Autodesk Inventor part; units mm, degrees
ref_plane "YZ Plane" through (0, 0, 0) normal (1, 0, 0) x (0, 1, 0)
ref_plane "XZ Plane" through (0, 0, 0) normal (0, 1, 0) x (-1, 0, 0)
ref_plane "XY Plane" through (0, 0, 0) normal (0, 0, 1) x (1, 0, 0)
sketch "Sketch1" plane through (0, 0, 0) normal (0, 1, 0) x (-1, 0, 0)
  circle A0 centre (0, 0) radius 3.1369
  dimension "d0" = 6.2738
extrude "Extrusion1" add sketch "Sketch1" along normal mid plane 6.35
sketch "Sketch2" plane through (0, 3.175, 0) normal (0, 1, 0) x (1, 0, 0)
  circle A0 centre (0, 0) radius 4.699
  dimension "d3" = 9.398
extrude "Extrusion2" add sketch "Sketch2" along normal blind 6.35
sketch "Sketch3" plane through (0, -3.175, 0) normal (0, -1, 0) x (1, 0, 0)
  circle A0 centre (0, 0) radius 3.1369
extrude "Extrusion3" add sketch "Sketch3" along normal blind 12.7
thread "Thread1"
sketch "Sketch4" plane through (0, 9.525, 0) normal (0, 1, 0) x (1, 0, 0)
  line L0 (0, -3.6955) -> (-3.2004, -1.8478)
  line L1 (-3.2004, -1.8478) -> (-3.2004, 1.8478)
  line L2 (-3.2004, 1.8478) -> (0, 3.6955)
  line L3 (0, 3.6955) -> (3.2004, 1.8478)
  line L4 (3.2004, 1.8478) -> (3.2004, -1.8478)
  line L5 (3.2004, -1.8478) -> (0, -3.6955)
  point P0 (0, 0)
  point P1 (0, 0)
  dimension "d10" = 6.4008
extrude "Extrusion4" cut sketch "Sketch4" against normal blind 3.81
properties part number "Bolt 2.0" material "Steel, Galvanized"
The listing builds one solid part. Answer for the finished solid, in the listing's coordinates (mm). A direction names the side the tool comes from. Give positions to 0.01 mm unless a question says otherwise; leave off trailing zeros. Write each loop counter-clockwise with the first axis right and the second up, starting at its lowest first coordinate (ties: lowest second). Pieces come first, ordered by that corner, then holes.
Item 1: Section A-A, the plane x = 2.25 is taken. Write down the section's boundary in (y, z) (1 decimal), plus the area to 3 significant figures.
Item 2: Section C-C, the plane y = 5 is taken. Write down the section's boundary in (x, z), plus the area to 3 significant figures.
Item 3: Determine the mould class of faces 4 (the flat face through (0, -15.875, 0)), 5 (the cylindrical face through (-0.61, 6.31, 4.66)), 6 (the flat face through (-1.578, 7.647, 2.785)) for opening direction Z: released by +Z, released by -Z, zero draft, split by the parting line, or undercut.
Item 4: Section B-B, the plane z = 0.75 is taken. Write down the section's boundary in (x, y) (3 decimals).
Item 5: Which of the six approach directions +Z, -Z, +X, -X, +Y, -Y give full straight-line access (tool end or side, diameter ignored) to faces 1 (the flat face through (1.578, 7.647, -2.785)), 2 (the flat face through (2, 9.525, 3)), 3 (the flat face through (-1.1, 3.175, 3.1))?
Item 6: Section D-D, the plane y = -12.75 is taken. Write down the section's boundary in (x, z), plus the area to 3 significant figures.
Item 7: Flat-ended cylindrical pins translate along their axes: P1, Ø1.9, axis at x = -1.5, z = 1.5, coming from the +Y side (3 decimals); P2, Ø1, axis at y = -12, z = -2, coming from the -X side (3 decimals); P3, Ø2, axis at y = -12, z = -2, coming from the -X side. Find the tip coordinate at first contact, or state that the pin passes through.
Item 8: Find the intervals of material crossed by line 1 along Y through (x, z) = (0, -3.25) (3 decimals); line 2 along X through (y, z) = (-5.25, 0); line 3 along Y through (x, z) = (3, 2.25) (3 decimals), in increasing order.
Completed:
1. outline: (-15.9, -2.2) - (3.2, -2.2) - (3.2, -4.1) - (9.5, -4.1) - (9.5, -2.4) - (5.7, -2.4) - (5.7, 2.4) - (9.5, 2.4) - (9.5, 4.1) - (3.2, 4.1) - (3.2, 2.2) - (-15.9, 2.2) - close
1. area: 117 mm2
2. outline: circle Ø9.4 at (0, 0)
2. area: 69.4 mm2
3. face 4: zero draft
3. face 5: split by the parting line
3. face 6: undercut
4. outline: (-4.639, 3.175) - (-3.046, 3.175) - (-3.046, -15.875) - (3.046, -15.875) - (3.046, 3.175) - (4.639, 3.175) - (4.639, 9.525) - (3.2, 9.525) - (3.2, 5.715) - (-3.2, 5.715) - (-3.2, 9.525) - (-4.639, 9.525) - close
5. face 1: +Y
5. face 2: +Z, -Z, +X, -X, +Y
5. face 3: -Y
6. outline: circle Ø6.27 at (0, 0)
6. area: 30.9 mm2
7. P1: stops at y = 5.715
7. P2: stops at x = -2.755
7. P3: stops at x = -2.97
8. line 1: y = 3.175 to 5.715
8. line 2: x = -3.14 to 3.14
8. line 3: y = 3.175 to 9.525
